Source: CAD feature listing. Evaluate the final solid. Frame: model axes, mm. Face numbers are marked on the shaded views. Coordinates: 2 decimals unless noted, no trailing zeros. Loops run counter-clockwise (first coordinate to the right, second up) from the corner with the lowest first, then second, coordinate; pieces in that order, holes last. Notation, with made-up numbers: M -31,-10.5 L 1,-10.5 A21 cw 1,10.5 Z; hole C 76.25,-26 d3. An arc over 180 degrees is marked long. Write each question's results on one line, items separated by ' | '. Start each with the question number.
from build123d import *

# Parameters (mm, degrees)
F0_R      = 60
F1_DEPTH  = 20
F3_DEPTH  = 10
F4_W      = 5
F4_H      = 70
F5_DEPTH  = 60
F7_DEPTH  = 3
F8_W      = 11.8
F8_H      = 22.5
F9_DEPTH  = 6
F10_W     = 5
F10_H     = 1.5
F10_W_2   = 2.5
F10_H_2   = 1
F10_W_3   = 7.5
F11_DEPTH = 16
F12_W     = 10
F12_H     = 8
F13_DEPTH = 20.001


with BuildPart() as f1:
    # F0 (on Front) → F1 (new body)
    with BuildSketch(Plane.XZ):
        Circle(F0_R)
    extrude(amount=F1_DEPTH)

    # F2 (on face) → F3 (cut)
    with BuildSketch(Plane.XZ.offset(20)):
        with BuildLine():
            Line((-25, -12.5), (-25, 12.5))
            Line((-25, 12.5), (-58.6834729715, 12.5))
            ThreePointArc((-58.6834729715, 12.5), (-59.6699605258, 6.2845692656), (-60, 0))
            ThreePointArc((-60, 0), (-59.6699605258, -6.2845692656), (-58.6834729715, -12.5))
            Line((-58.6834729715, -12.5), (-25, -12.5))
        make_face()
        with BuildLine():
            Line((58.6834729715, 12.5), (25, 12.5))
            Line((25, 12.5), (25, -12.5))
            Line((25, -12.5), (58.6834729715, -12.5))
            ThreePointArc((58.6834729715, -12.5), (59.6699605258, -6.2845692656), (60, 0))
            ThreePointArc((60, 0), (59.6699605258, 6.2845692656), (58.6834729715, 12.5))
        make_face()
    extrude(amount=-F3_DEPTH, mode=Mode.SUBTRACT)

    # F4 (on Right) → F5 (cut, symmetric)
    with BuildSketch(Plane.YZ):
        with Locations((-12.5, 0)):
            Rectangle(F4_W, F4_H)
    extrude(amount=F5_DEPTH, both=True, mode=Mode.SUBTRACT)

    # F6 (on face) → F7 (cut)
    with BuildSketch(Plane.XZ.offset(10)):
        with BuildLine():
            Line((30, -22.5), (30, -25))
            Line((30, -25), (-30, -25))
            Line((-30, -25), (-30, -22.5))
            Line((-30, -22.5), (-55.6214886532, -22.5))
            ThreePointArc((-55.6214886532, -22.5), (-54.531492065, -25.0263136152), (-53.3268225193, -27.5))
            Line((-53.3268225193, -27.5), (0, -27.5))
            Line((0, -27.5), (53.3268225193, -27.5))
            ThreePointArc((53.3268225193, -27.5), (54.531492065, -25.0263136152), (55.6214886532, -22.5))
            Line((55.6214886532, -22.5), (30, -22.5))
        make_face()
        with BuildLine():
            Line((30, 25), (30, 22.5))
            Line((30, 22.5), (55.6214886532, 22.5))
            ThreePointArc((55.6214886532, 22.5), (54.531492065, 25.0263136152), (53.3268225193, 27.5))
            Line((53.3268225193, 27.5), (0, 27.5))
            Line((0, 27.5), (-53.3268225193, 27.5))
            ThreePointArc((-53.3268225193, 27.5), (-54.531492065, 25.0263136152), (-55.6214886532, 22.5))
            Line((-55.6214886532, 22.5), (-30, 22.5))
            Line((-30, 22.5), (-30, 25))
            Line((-30, 25), (30, 25))
        make_face()
        Polygon((0, 22.5), (30, 22.5), (30, 25), (-30, 25), (-30, 22.5), align=None)
        Polygon((-30, -25), (30, -25), (30, -22.5), (0, -22.5), (-30, -22.5), align=None)
    extrude(amount=-F7_DEPTH, mode=Mode.SUBTRACT)

    # F8 (on face) → F9 (cut)
    with BuildSketch(Plane.XZ.offset(20)):
        with Locations((0, -5.35)):
            Rectangle(F8_W, F8_H)
    extrude(amount=-F9_DEPTH, mode=Mode.SUBTRACT)

    # F10 (on face) → F11 (cut)
    with BuildSketch(Plane.XZ.offset(20)):
        with Locations((-35, 26.75)):
            Rectangle(F10_W, F10_H)
        with Locations((-33.75, 24.5)):
            Rectangle(F10_W_2, F10_H_2)
        with Locations((35, 26.75)):
            Rectangle(F10_W, F10_H)
        with Locations((33.75, 24.5)):
            Rectangle(F10_W_2, F10_H_2)
        with Locations((35, -26.75)):
            Rectangle(F10_W, F10_H)
        with Locations((33.75, -24.5)):
            Rectangle(F10_W_2, F10_H_2)
        with Locations((-35, -26.75)):
            Rectangle(F10_W, F10_H)
        with Locations((-33.75, -24.5)):
            Rectangle(F10_W_2, F10_H_2)
        Polygon((32.5, 25), (35, 25), (35, 24), (37.5, 24), (37.5, 26), (32.5, 26), align=None)
        with Locations((36.25, 23.25)):
            Rectangle(F10_W_2, F10_H)
        with Locations((33.75, 23.25)):
            Rectangle(F10_W_2, F10_H)
        with Locations((28.75, 24.5)):
            Rectangle(F10_W_3, F10_H_2)
        with Locations((28.75, 25.5)):
            Rectangle(F10_W_3, F10_H_2)
        Polygon((-35, -25), (-35, -24), (-37.5, -24), (-37.5, -26), (-32.5, -26), (-32.5, -25), align=None)
        with Locations((-33.75, -23.25)):
            Rectangle(F10_W_2, F10_H)
        with Locations((-36.25, -23.25)):
            Rectangle(F10_W_2, F10_H)
        with Locations((-28.75, -24.5)):
            Rectangle(F10_W_3, F10_H_2)
        with Locations((-28.75, -25.5)):
            Rectangle(F10_W_3, F10_H_2)
        Polygon((37.5, -24), (35, -24), (35, -25), (32.5, -25), (32.5, -26), (37.5, -26), align=None)
        with Locations((36.25, -23.25)):
            Rectangle(F10_W_2, F10_H)
        with Locations((33.75, -23.25)):
            Rectangle(F10_W_2, F10_H)
        Polygon((-35, 25), (-32.5, 25), (-32.5, 26), (-37.5, 26), (-37.5, 24), (-35, 24), align=None)
        with Locations((-36.25, 23.25)):
            Rectangle(F10_W_2, F10_H)
        with Locations((-33.75, 23.25)):
            Rectangle(F10_W_2, F10_H)
        with Locations((-28.75, 25.5)):
            Rectangle(F10_W_3, F10_H_2)
        with Locations((-28.75, 24.5)):
            Rectangle(F10_W_3, F10_H_2)
        with Locations((28.75, -25.5)):
            Rectangle(F10_W_3, F10_H_2)
        with Locations((28.75, -24.5)):
            Rectangle(F10_W_3, F10_H_2)
    extrude(amount=-F11_DEPTH, mode=Mode.SUBTRACT)

    # F12 (on face) → F13 (cut, through all)
    with BuildSketch(Plane.XZ.offset(20)):
        with Locations((0, -46.5785360177)):
            Rectangle(F12_W, F12_H)
    extrude(amount=-F13_DEPTH, mode=Mode.SUBTRACT)


solid = f1.part
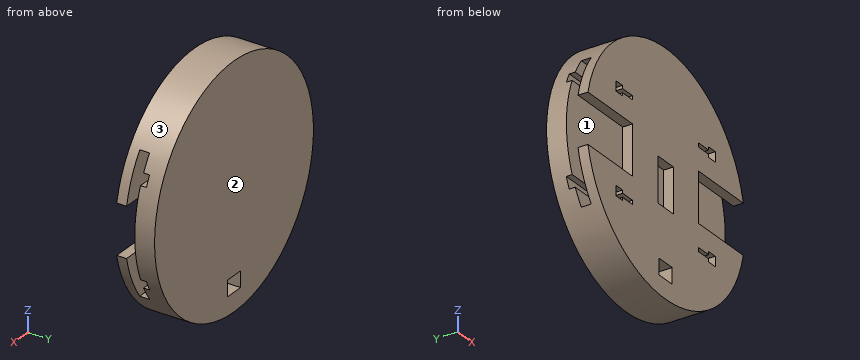
Item 1: Cut plane A-A (y = -12.75). Output: boundary loops of the cut face in (x, z).
Item 2: First-contact query: pin 1 Ø1.8 at (x, y) = (-0.5, -8.5) entering from +Z; pin 2 Ø1.5 at (x, z) = (-33.5, -24) entering from -Y; pin 3 Ø12 at (y, z) = (-5, -36) entering from -X. Flat tips, straight axial feed; report the tip coordinate or a pass-through.
Item 3: Mould query, pull axis Z, two halves, no side actions, for the marked faces 1, 2 and 3. Classes: +Z half, -Z half, draft (parallel to the pull), parting line (faces both ways), or undercut.
Item 4: Cut plane C-C (x = 0). Output: boundary loops of the cut face in (y, z).
Item 5: Cut plane D-D (y = -2.5). Output: boundary loops of the cut face in (x, z), then the cut area to 3 significant figures.
Item 6: Cut plane B-B (z = 0). Output: boundary loops of the cut face in (x, y).
Item 7: Line query: probe 1 along Z at (x, y) = (-0.5, -13.5); probe 2 along Y at (x, z) = (-8.5, 10); probe 3 along Y at (x, z) = (-33, -23). Output: solid intervals per line, ascending.
Response values:
1) outline: M -48.73,-35 A60 ccw 48.73,-35 Z; M -48.73,35 L 48.73,35 A60 ccw Z; hole M -5,-50.58 L 5,-50.58 L 5,-42.58 L -5,-42.58 Z
2) pin 1: stops at z = 60 | pin 2: stops at y = -4 | pin 3: stops at x = -51.96
3) face 1: undercut | face 2: draft | face 3: parting line
4) outline: M -20,-60 L 0,-60 L 0,-50.58 L -20,-50.58 Z; M -20,-42.58 L 0,-42.58 L 0,60 L -20,60 L -20,5.9 L -15,5.9 L -15,35 L -10,35 L -10,27.5 L -7,27.5 L -7,22.5 L -10,22.5 L -10,-22.5 L -7,-22.5 L -7,-27.5 L -10,-27.5 L -10,-35 L -15,-35 L -15,-16.6 L -20,-16.6 Z
5) outline: C 0,0 d120; hole M -5,-50.58 L 5,-50.58 L 5,-42.58 L -5,-42.58 Z | area: 11,200 mm2
6) outline: M -60,-10 L 60,-10 L 60,0 L -60,0 Z; M -25,-20 L -5.9,-20 L -5.9,-15 L -25,-15 Z; M 5.9,-20 L 25,-20 L 25,-15 L 5.9,-15 Z
7) probe 1: z = -60 to -50.58, -42.58 to -35, 35 to 60 | probe 2: y = -20 to -15, -10 to 0 | probe 3: y = -4 to 0
